Verification items for the finished model (mm, model axes). A direction names the side the tool comes from. Give positions to 0.01 mm unless a question says otherwise; leave off trailing zeros. Write each loop counter-clockwise with the first axis right and the second up, starting at its lowest first coordinate (ties: lowest second). Pieces come first, ordered by that corner, then holes. Notation, with made-up numbers: (81, 35.5) - (135, 35.5) arc R9 cw to (135, 50.5) - close; hole circle Ø8 at (86, 87.25). An arc over 180 degrees is marked (long way). Answer as a JSON object with one key per item and string values. Group by question number.
Item 1: Sectioned sample at B-B, the plane z = 1.75. Record the boundary of the cut face in (x, y), and give its area (3 significant figures).
Item 2: Sectioned sample at D-D, the plane z = 8.5. Record the boundary of the cut face in (x, y).
Item 3: Draft check along X on faces 1 (the face through (10, -6.062, 2)), 2 (the face through (4.726, -2.989, 2.465)), 3 (the face through (0, 10, 5)), 4 (the face through (-20, 0, 5)). Enter one of: +X half, -X half, draft (parallel to the pull), parting line (faces both ways), or undercut.
Item 4: Sectioned sample at A-A, the plane x = 10. Record the boundary of the cut face in (y, z), and give its area (3 significant figures).
Item 5: Go/stop test with flat-tipped pins: pin 1 (0.6 mm diameter, centred on x = -9, y = -5, fed in from -Z); pin 2 (3 mm diameter, centred on x = -7, y = -1.5, fed in from -Z). Record where each tip stops, or that it passes through.
Item 6: Scan lines: line 1 along Y through (x, z) = (10, 6.6); line 2 along X through (y, z) = (3.25, 7); line 3 along Y through (x, z) = (-9, 4.75). Record each from-to range of solid material in increasing order. Write a range as [from, to].
Item 7: Tool access check on faces 5 (the face through (6, 0, 7)), 6 (the face through (-4, 3, 5)), 7 (the face through (4.774, 3.074, 2.465)). Record the directions out of +Z, -Z, +X, -X, +Y, -Y that give a thin tool (end or side, any length) a straight path to the whole face; none if there is none.
```python
from build123d import *

# Parameters (mm, degrees)
SKETCH_W        = 40
SKETCH_H        = 20
SKETCH_R        = 4
PAD_DEPTH       = 10
POCKET_DEPTH    = 5
SKETCH002_W     = 14
SKETCH002_H     = 8
POCKET001_DEPTH = 0.2
SKETCH003_W     = 8
SKETCH003_H     = 8
POCKET002_DEPTH = 0.2


with BuildPart() as part:
    # Sketch → Pad (new body)
    with BuildSketch(Plane.XY):
        Rectangle(SKETCH_W, SKETCH_H)
        with Locations((-10, 0)):
            Circle(SKETCH_R, mode=Mode.SUBTRACT)
        with Locations((10, 0)):
            Circle(SKETCH_R, mode=Mode.SUBTRACT)
    extrude(amount=PAD_DEPTH)

    # Sketch001 → Pocket (cut)
    with BuildSketch(Plane.XY):
        Polygon((-6.5, 6.062178), (-13.5, 6.062178), (-17, 0), (-13.5, -6.062178), (-6.5, -6.062178), (-3, 0), align=None)
        Polygon((13.5, 6.062178), (6.5, 6.062178), (3, 0), (6.5, -6.062178), (13.5, -6.062178), (17, 0), align=None)
    extrude(amount=POCKET_DEPTH, mode=Mode.SUBTRACT)

    # Sketch002 (on Face21 of Pocket) → Pocket001 (cut)
    with BuildSketch(Plane(origin=(0, 0, 5), x_dir=(1, 0, 0), z_dir=(0, 0, -1))):
        with Locations((-10, 0)):
            Rectangle(SKETCH002_W, SKETCH002_H)
    extrude(amount=-POCKET001_DEPTH, mode=Mode.SUBTRACT)

    # Sketch003 (on Face28 of Pocket001) → Pocket002 (cut)
    with BuildSketch(Plane(origin=(0, 0, 5.2), x_dir=(1, 0, 0), z_dir=(0, 0, -1))):
        with Locations((-10, 0)):
            Rectangle(SKETCH003_W, SKETCH003_H)
    extrude(amount=-POCKET002_DEPTH, mode=Mode.SUBTRACT)


solid = part.part
```
Geometry check:
{
 "1": {"outline": "(-20, -10) - (20, -10) - (20, 10) - (-20, 10) - close; hole (-17, 0) - (-13.5, -6.06) - (-6.5, -6.06) - (-3, 0) - (-6.5, 6.06) - (-13.5, 6.06) - close; hole (3, 0) - (6.5, -6.06) - (13.5, -6.06) - (17, 0) - (13.5, 6.06) - (6.5, 6.06) - close", "area": "545 mm^2"},
 "2": {"outline": "(-20, -10) - (20, -10) - (20, 10) - (-20, 10) - close; hole circle Ø8 at (-10, 0); hole circle Ø8 at (10, 0)"},
 "3": {"face 1": "undercut", "face 2": "undercut", "face 3": "draft", "face 4": "-X half"},
 "4": {"outline": "(-10, 0) - (-6.06, 0) - (-6.06, 5) - (-4, 5) - (-4, 10) - (-10, 10) - close; (4, 5) - (6.06, 5) - (6.06, 0) - (10, 0) - (10, 10) - (4, 10) - close", "area": "99.4 mm^2"},
 "5": {"pin 1": "z = 5", "pin 2": "z = 5.2"},
 "6": {"line 1": "[-10, -4], [4, 10]", "line 2": "[-20, -12.33], [-7.67, 7.67], [12.33, 20]", "line 3": "[-10, -6.06], [6.06, 10]"},
 "7": {"face 5": "+Z, -Z", "face 6": "none", "face 7": "-Z"}
}
